Autodesk Inventor part; units mm, degrees
ref_plane "YZ Plane" through (0, 0, 0) normal (1, 0, 0) x (0, 1, 0)
ref_plane "XZ Plane" through (0, 0, 0) normal (0, 1, 0) x (-1, 0, 0)
ref_plane "XY Plane" through (0, 0, 0) normal (0, 0, 1) x (1, 0, 0)
sketch "Sketch1" plane through (0, 0, 0) normal (1, 0, 0) x (0, 1, 0)
  line L0 (30, 0) -> (30, -55)
  line L1 (30, -55) -> (20, -55)
  line L2 (20, -55) -> (20, -45)
  line L3 (20, -45) -> (0, -45)
  line L4 (0, -45) -> (0, -10)
  line L5 (0, -10) -> (20, -10)
  line L6 (20, -10) -> (20, 0)
  line L7 (20, 0) -> (30, 0)
  point P0 (0, 0)
  dimension "d0" = 55
  dimension "d1" = 10
  dimension "d2" = 10
  dimension "d3" = 20
  dimension "d4" = 35
  dimension "d5" = 20
  dimension "d6" = 10
  dimension "d7" = 30
  dimension "d8" = 0
extrude "Extrusion1" add sketch "Sketch1" against normal blind 140
sketch "Sketch3" plane through (0, 0, 0) normal (1, 0, 0) x (0, 0, -1)
  line L0 (55, 30) -> (0, 30)
  line L1 (10, 20) -> (10, 0)
  line L2 (45, 0) -> (45, 20)
  line L3 (10, 0) -> (45, 0)
  point P0 (0, 0)
  point P1 (17, 23)
  point P2 (38, 23)
  point P3 (17, 7)
  point P4 (38, 7)
  dimension "d26" = 7
  dimension "d27" = 7
  dimension "d28" = 7
  dimension "d29" = 7
  dimension "d30" = 7
  dimension "d31" = 7
  dimension "d32" = 7
  dimension "d33" = 7
hole "Hole2" at (0, 23, -17) at (0, 23, -38) at (0, 7, -38) at (0, 7, -17) direction (-1, 0, 0) diameter 4.917 depth 20 tip angle 118 counterbore diameter 6 counterbore depth 15
sketch "Sketch4" plane through (-140, 0, 0) normal (-1, 0, 0) x (0, 0, 1)
  line L0 (-45, 0) -> (-10, 0)
  line L1 (-45, 20) -> (-45, 0)
  line L2 (-10, 0) -> (-10, 20)
  point P0 (0, 0)
  point P1 (-38, 23)
  point P2 (-17, 23)
  point P3 (-27.6865, 8)
  dimension "d41" = 8
  dimension "d42" = 23
  dimension "d43" = 23
  dimension "d44" = 7
  dimension "d45" = 7
hole "Hole3" at (-140, 8, -27.6865) at (-140, 23, -38) at (-140, 23, -17) direction (1, 0, 0) diameter 4.917 depth 20 tip angle 118 counterbore diameter 6 counterbore depth 15
sketch "Sketch5" plane through (0, 0, -45) normal (0, -1, 0) x (1, 0, 0)
  line L0 (0, 35) -> (0, 0)
  line L1 (0, 45) -> (-140, 45)
  line L2 (0, -10) -> (-140, -10)
  point P0 (-115, 30)
  point P1 (-70, 30)
  point P2 (-25, 30)
  point P3 (-115, 5)
  point P4 (-70, 5)
  point P5 (-25, 5)
  dimension "d53" = 25
  dimension "d61" = 25
  dimension "d62" = 15
  dimension "d63" = 15
  dimension "d64" = 15
  dimension "d65" = 15
  dimension "d66" = 15
  dimension "d67" = 15
  dimension "d68" = 45
  dimension "d69" = 45
  dimension "d70" = 45
  dimension "d71" = 45
hole "Hole4" at (-115, 0, -15) at (-70, 0, -15) at (-115, 0, -40) at (-70, 0, -40) at (-25, 0, -40) at (-25, 0, -15) direction (0, 1, 0) diameter 5.134 depth 16.2 tip angle 118
properties part number "Fuhrung" material "Steel, Mild"
Geometry: final body of the model. Coordinates: model frame, mm. A direction names the side the tool comes from. Round coordinates to 2 decimals unless told otherwise and drop trailing zeros. Write each loop counter-clockwise with the first axis right and the second up, starting at its lowest first coordinate (ties: lowest second). Pieces come first, ordered by that corner, then holes. Notation, with made-up numbers: M 18.5,-32 L 49.5,-32 A23 cw 49.5,2 Z; hole C -1.75,-30.5 d6. An arc over 180 degrees is marked long. Answer in a Markdown table with one row per item. Add a question column.
(1) Ray query, L1, parallel to Z at x = -25, y = 5; L2, parallel to Z at x = -8.5, y = 7; L3, parallel to X at y = 13, z = -40. Return the intervals inside material, ascending.
(2) Reachability of faces 5 (the face through (-71.735, 8.213, -13.108)), 6 (the face through (-17.54, 7.94, -40.27)), 7 (the face through (-69, 10, -45)) from +Z, -Z, +X, -X, +Y, -Y: full face, straight path, thin tool, end or side. Return the list, or none.
(3) Contact query for flat-ended pins moving along their axis: pin 1 (3 mm diameter, centred on x = -77.5, y = 9.5, fed in from +Z); pin 2 (3 mm diameter, centred on y = 23, z = -17, fed in from +X); pin 3 (8 mm diameter, centred on x = -103, y = 4.5, fed in from -Z). Output: stop coordinate, or through.
(4) Cut plane B-B, the plane z = -49. Return the cut outline in (x, y), then the cut area to 3 significant figures.
(5) Draft query along X for faces 1 (the face through (-69, 20, -50)), 2 (the face through (-25.44, 17.47, -14.9)), 3 (the face through (-117.165, 8.213, -41.38)), 4 (the face through (-140, 18, -27)). Return one class per face: pulls with the +X half, pulls with the -X half, needs draft (parallel to the pull), parting line crosses it, or undercut.
(6) Cut plane A-A, the plane x = -98. Return the cut outline in (y, z), then the cut area to 3 significant figures.
Established:
| question | item | result |
|---|---|---|
| 1 | L1 | -45 to -42.57, -37.43 to -17.57, -12.43 to -10 |
| 1 | L2 | -45 to -41, -35 to -20, -14 to -10 |
| 1 | L3 | -140 to -117.57, -112.43 to -72.57, -67.43 to -27.57, -22.43 to 0 |
| 2 | face 5 | -Y |
| 2 | face 6 | +X |
| 2 | face 7 | -Z, +X, -X, -Y |
| 3 | pin 1 | z = -10 |
| 3 | pin 2 | x = -20.58 |
| 3 | pin 3 | z = -45 |
| 4 | outline | M -140,20 L 0,20 L 0,30 L -140,30 Z |
| 4 | area | 1,400 mm² |
| 5 | face 1 | needs draft |
| 5 | face 2 | undercut |
| 5 | face 3 | undercut |
| 5 | face 4 | pulls with the -X half |
| 6 | outline | M 0,-45 L 20,-45 L 20,-55 L 30,-55 L 30,0 L 20,0 L 20,-10 L 0,-10 Z |
| 6 | area | 1,250 mm² |
